Autodesk Inventor part; units mm, degrees
ref_plane "Work Plane1" through (4.25, 0, 0) normal (0, 0, -1) x (1, 0, 0)
ref_plane "YZ Plane" through (0, 0, 0) normal (1, 0, 0) x (0, 1, 0)
ref_plane "XZ Plane" through (0, 0, 0) normal (0, 1, 0) x (-1, 0, 0)
sketch "Sketch1" plane through (0, 0, 0) normal (0, 0, 1) x (1, 0, 0)
  line L0 (0, 0) -> (8, 0)
  line L1 (8, 0) -> (8, 1)
  line L2 (8, 1) -> (0.5, 1)
  line L3 (0.5, 1) -> (0, 0.5)
  line L4 (0, -0.2) -> (0, 1.2)
  line L5 (0, 0.5) -> (0.2887, 0)
  line L6 (0, 1.2) -> (0, -0.2)
  dimension "d0" = 2
  dimension "d2" = 8
  dimension "d3" = 45
  dimension "d4" = 1
  dimension "d14" = 60
revolve "Body" add sketch "Sketch1" angle 360 about axis through (0, 0, 0) along (1, 0, 0) contours L5 L3 L2 L1 L0
chamfer "Chamfer1" distance 0.2454 angle 45 1 edges at (8, -1, 0) measured on face at (8, 0.2495, 0.221)
sketch "Sketch2" plane through (0, 0, 0) normal (0, 0, 1) x (1, 0, 0)
  line L0 (8, 0.7546) -> (8, -0.7546)
  line L1 (7.232, 0) -> (8.128, 0)
  line L2 (8, 0.125) -> (7.36, 0.125)
  line L3 (7.36, 0.125) -> (7.36, 0)
  line L4 (7.36, -0.125) -> (7.36, 0)
  line L5 (7.36, -0.125) -> (8, -0.125)
  dimension "d10" = 0.125
  dimension "d11" = 0.64
extrude "Slot" cut sketch "Sketch2" against normal mid plane 2
thread "Thread"
ref_plane "Work Plane1" through (4.25, 0, 0) normal (0, 0, -1) x (1, 0, 0)
equation "\"d10\" = 0.5 * SBR"
equation "\"d11\" = STI"
equation "\"d12\" = NND"
equation "\"d5\" = -0.5 * GD1 + 0.5 * NND"
equation "\"d7\" = FAWI"
equation "\"d34\" = -0.5 * GD1 + 0.5 * NND"
equation "\"d8\" = NLG"
equation "\"d0\" = NND"
equation "\"d2\" = NLG"
equation "\"d3\" = FAWI1"
equation "\"d4\" = SPD"
equation "\"d14\" = 0.5 * ANG"
equation "\"NND\" = 2"
equation "\"NLG\" = 8"
equation "\"FAWI\" = 45deg"
equation "\"GD1\" = THREADDIA - 1.2269 * PTC"
equation "\"FAWI1\" = 45deg"
equation "\"SPD\" = 1"
equation "\"SBR\" = 0.25"
equation "\"STI\" = 0.64"
equation "\"ANG\" = 120deg"
equation "\"GUL\" = 0.61345 * PTC"
equation "\"THREADDIA\" = 2"
equation "\"TOA\" = 30deg"
equation "\"PTC\" = 0.4"
equation "\"GAL\" = 0.61345 * PTC"
properties part number "ISO 7436 - M2 x 8" material "Stainless Steel, 440C"
Geometry check sheet. Reference: the model listing, model coordinates, mm. Round coordinates to 2 decimals unless told otherwise and drop trailing zeros. Order: outer loops, then holes, each group sorted by start corner. A loop starts at its lowest first (then second) coordinate and runs counter-clockwise, first axis right, second up. Notation, with made-up numbers: M -7,27 L 7,27 A19 cw 7,58 Z; hole C 25.25,-2.5 d2. An arc over 180 degrees is marked long. Answer as CSV lines item,"result".
1) Gauge pin test, flat ends, axial feed: pin 1 Ø0.7 at (x, z) = (8, 0.5) entering from -Y; pin 2 Ø1 at (x, y) = (4.5, -0.5) entering from +Z. Record the tip position at first contact, or that the pin passes through.
Entries:
pin 1,"y = -0.97"
pin 2,"z = 1"
2) Sectioned sample at A-A on x = 5. Record the cut outline in (y, z), and give its area (3 significant figures).
Entries:
outline,"C 0,0 d2"
area,"3.14 mm2"
3) Thickness scan on probe 1 along X at (y, z) = (0.45, -0.8); probe 2 along Z at (x, y) = (1.25, 0.35); probe 3 along X at (y, z) = (-0.6, 0.5). Record the ranges inside material, lowest first. Write a range as [from, to].
Entries:
probe 1,"[0.42, 7.84]"
probe 2,"[-0.94, 0.94]"
probe 3,"[0.28, 7.97]"
4) Mould release check, pull along Y, two halves, no side actions. Record for faces 1 (the face through (0.24, -0.06, -0.06)), 2 (the face through (7.876, 0.879, 0.018)), 3 (the face through (4, 0, 1)): +Y half, -Y half, draft (parallel to the pull), parting line (faces both ways), or undercut.
Entries:
face 1,"undercut"
face 2,"+Y half"
face 3,"parting line"
